```python
from build123d import *

# Parameters (mm, degrees)
SKETCH_1_R          = 10
EXTRUDE_1_DEPTH     = 3
SKETCH_2_R          = 6
EXTRUDE_2_DEPTH     = 20
CUT_EXTRUDE_1_REACH = 29
SKETCH_4_R          = 1.25


with BuildPart() as part:
    # 草图1 → 凸台-拉伸1 (new body)
    with BuildSketch(Plane.XY):
        Circle(SKETCH_1_R)
    extrude(amount=EXTRUDE_1_DEPTH)

    # 草图2 → 凸台-拉伸2 (add)
    with BuildSketch(Plane.XY.offset(3)):
        Circle(SKETCH_2_R)
    extrude(amount=EXTRUDE_2_DEPTH)

    # 草图4 → 切除-拉伸1 (cut, up to next)
    with BuildSketch(Plane(origin=(0, 0, 0), x_dir=(-1, 0, 0), z_dir=(0, 0, -1)), mode=Mode.PRIVATE) as cut_extrude_1_sk1:
        with Locations((-5.303300859, 5.303300859)):
            Circle(SKETCH_4_R)
    cut_extrude_1_tool1 = extrude(cut_extrude_1_sk1.sketch, amount=-CUT_EXTRUDE_1_REACH, mode=Mode.PRIVATE) & part.part
    # 草图4 → 切除-拉伸1 (cut, up to next)
    with BuildSketch(Plane(origin=(0, 0, 0), x_dir=(-1, 0, 0), z_dir=(0, 0, -1)), mode=Mode.PRIVATE) as cut_extrude_1_sk2:
        with Locations((5.303300859, 5.303300859)):
            Circle(SKETCH_4_R)
    cut_extrude_1_tool2 = extrude(cut_extrude_1_sk2.sketch, amount=-CUT_EXTRUDE_1_REACH, mode=Mode.PRIVATE) & part.part
    # 草图4 → 切除-拉伸1 (cut, up to next)
    with BuildSketch(Plane(origin=(0, 0, 0), x_dir=(-1, 0, 0), z_dir=(0, 0, -1)), mode=Mode.PRIVATE) as cut_extrude_1_sk3:
        with Locations((5.303300859, -5.303300859)):
            Circle(SKETCH_4_R)
    cut_extrude_1_tool3 = extrude(cut_extrude_1_sk3.sketch, amount=-CUT_EXTRUDE_1_REACH, mode=Mode.PRIVATE) & part.part
    # 草图4 → 切除-拉伸1 (cut, up to next)
    with BuildSketch(Plane(origin=(0, 0, 0), x_dir=(-1, 0, 0), z_dir=(0, 0, -1)), mode=Mode.PRIVATE) as cut_extrude_1_sk4:
        with Locations((-5.303300859, -5.303300859)):
            Circle(SKETCH_4_R)
    cut_extrude_1_tool4 = extrude(cut_extrude_1_sk4.sketch, amount=-CUT_EXTRUDE_1_REACH, mode=Mode.PRIVATE) & part.part
    add(cut_extrude_1_tool1.solids().sort_by_distance((5.303301, 5.303301, 0))[0], mode=Mode.SUBTRACT)
    add(cut_extrude_1_tool2.solids().sort_by_distance((-5.303301, 5.303301, 0))[0], mode=Mode.SUBTRACT)
    add(cut_extrude_1_tool3.solids().sort_by_distance((-5.303301, -5.303301, 0))[0], mode=Mode.SUBTRACT)
    add(cut_extrude_1_tool4.solids().sort_by_distance((5.303301, -5.303301, 0))[0], mode=Mode.SUBTRACT)


solid = part.part
```
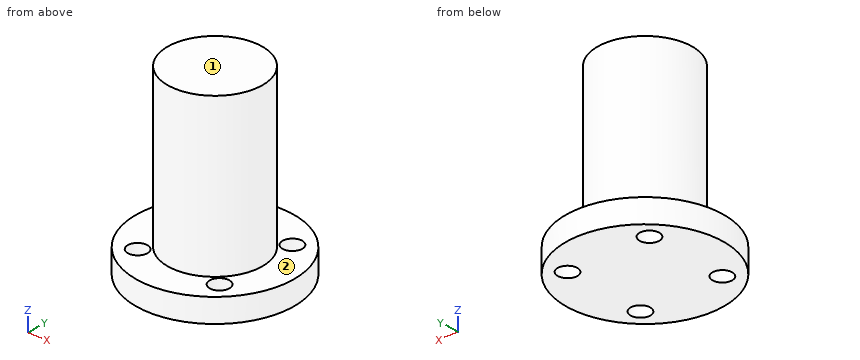
Here's how the part is built. I have some questions about the finished solid (model axes, mm). Face numbers are marked on the shaded views. A direction names the side the tool comes from. Round coordinates to 2 decimals unless told otherwise and drop trailing zeros. Order: outer loops, then holes, each group sorted by start corner. A loop starts at its lowest first (then second) coordinate and runs counter-clockwise, first axis right, second up. Notation, with made-up numbers: (4, -17) -> (52, -17) arc R22 ccw to (52, 16) -> close; hole circle Ø2 at (54, 57.5). An arc over 180 degrees is marked (long way). Use a Markdown table: item, result. Add a question column.
(1) Suppose I cut it at C-C, the plane z = 10.75. Please give me the cut outline in (x, y).
(2) I need wall thicknesses on line 1 along Y through (x, z) = (0.25, 14.75); line 2 along Z through (x, y) = (7.5, -0.25); line 3 along Y through (x, z) = (-3.5, 13). Which ranges of each line are inside material? Lowest first, please.
(3) Suppose I cut it at D-D, the plane y = -8. Please give me the cut outline in (x, z).
(4) For the marked faces 1 and 2, which set-ups out of +Z, -Z, +X, -X, +Y, -Y let a thin tool reach every point of the face, with its end or its side?
(5) For pin 1 Ø12 at (x, z) = (-6.5, 15) entering from +Y; pin 2 Ø8 at (y, z) = (1, 8) entering from +X; pin 3 Ø10 at (y, z) = (-8, 20.5) entering from -X; pin 4 Ø12 at (x, y) = (5, 6) entering from +Z, each with a flat end and sliding along its axis, tell me the tip position at first contact or that it passes through.
(6) Suppose I cut it at A-A, the plane y = 0. Please give me the cut outline in (x, z).
Verdict:
| question | item | result |
|---|---|---|
| 1 | outline | circle Ø12 at (0, 0) |
| 2 | line 1 | -5.99 to 5.99 |
| 2 | line 2 | 0 to 3 |
| 2 | line 3 | -4.87 to 4.87 |
| 3 | outline | (-6, 0) -> (6, 0) -> (6, 3) -> (-6, 3) -> close |
| 4 | face 1 | +Z, +X, -X, +Y, -Y |
| 4 | face 2 | +Z |
| 5 | pin 1 | y = 5.98 |
| 5 | pin 2 | x = 6 |
| 5 | pin 3 | x = -5.2 |
| 5 | pin 4 | z = 23 |
| 6 | outline | (-10, 0) -> (10, 0) -> (10, 3) -> (6, 3) -> (6, 23) -> (-6, 23) -> (-6, 3) -> (-10, 3) -> close |
